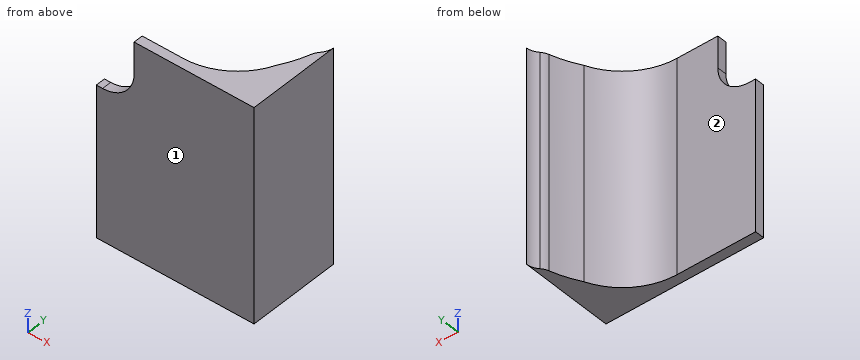
```python
from build123d import *

# Parameters (mm, degrees)
BOSS_EXTRUDE1_DEPTH = 68
CUT_EXTRUDE1_DEPTH  = 10


with BuildPart() as part:
    # Sketch2 → Boss-Extrude1 (new body)
    with BuildSketch(Plane.XY):
        with BuildLine():
            Line((-46.657067634, -11.60759921), (-71.613281954, -11.60759921))
            Line((-71.613281954, -11.60759921), (-71.613281954, -14.607279662))
            Line((-71.613281954, -14.607279662), (-21.613281954, -14.607279662))
            Line((-21.613281954, -14.607279662), (-21.613281954, 15.004436623))
            ThreePointArc((-21.613281954, 15.004436623), (-21.964992236, 13.162317544), (-22.970643034, 11.579355354))
            ThreePointArc((-22.970643034, 11.579355354), (-23.673981627, 10.626616994), (-24.133529038, 9.535190525))
            ThreePointArc((-24.133529038, 9.535190525), (-25.71874065, 5.128724796), (-27.866056136, 0.967129876))
            ThreePointArc((-27.866056136, 0.967129876), (-35.351914775, -8.173910524), (-46.657067634, -11.60759921))
        make_face()
    extrude(amount=BOSS_EXTRUDE1_DEPTH)

    # Sketch3 → Cut-Extrude1 (cut)
    with BuildSketch(Plane(origin=(0, -14.607279662, 0), x_dir=(-1, 0, 0), z_dir=(0, -1, 0))):
        with BuildLine():
            Line((71.613281954, -68), (59.613281954, -68))
            Line((59.613281954, -68), (59.613281954, -58))
            ThreePointArc((59.613281954, -58), (62.542214142, -50.928932188), (69.613281954, -48))
            Line((69.613281954, -48), (71.613281954, -48))
            Line((71.613281954, -48), (71.613281954, -68))
        make_face()
    extrude(amount=-CUT_EXTRUDE1_DEPTH, mode=Mode.SUBTRACT)


solid = part.part
```
Verification items for the finished model (mm, model axes). Face numbers are marked on the shaded views. A direction names the side the tool comes from. Coordinates: 2 decimals unless noted, no trailing zeros. Loops run counter-clockwise (first coordinate to the right, second up) from the corner with the lowest first, then second, coordinate; pieces in that order, holes last. Notation, with made-up numbers: (30, -20.5) -> (40, -20.5) arc R21 cw to (40, -14.5) -> close; hole circle Ø6 at (54.25, 28). An arc over 180 degrees is marked (long way). Answer in a Markdown table with one row per item. Add a question column.
1. Access from +Z, -Z, +X, -X, +Y, -Y to the whole of each face (thin tool, end or side, straight path). Record for the marked faces 1 and 2.
2. Section check A-A, the plane z = 49. Enter the section's corners in (x, y).
3. Section check D-D, the plane z = 8. Enter the section's corners in (x, y).
4. Section check B-B, the plane x = -55.5. Enter the section's corners in (y, z), then the cut area to 3 significant figures.
5. Depth check by flat-ended pin: P1, Ø12, axis at x = -66, z = 40, coming from the +Y side; P2, Ø1.5, axis at y = -7.5, z = 22.5, coming from the -X side; P3, Ø1.6, axis at x = -70.5, y = -12.5, coming from the +Z side. Enter the tip coordinate at first touch or a pass-through.
6. Section check C-C, the plane y = 1.75. Enter the section's corners in (x, z).
7. Material ranges on probe 1 along Y at (x, z) = (-55, 6.5); probe 2 along X at (y, z) = (-10, 34); probe 3 along X at (y, z) = (1, 22.5), recorded low to high. Write a range as [from, to].
Derived:
| question | item | result |
|---|---|---|
| 1 | face 1 | +Z, -Z, +X, -X, -Y |
| 1 | face 2 | +Z, -Z, -X, +Y |
| 2 | outline | (-65.25, -14.61) -> (-21.61, -14.61) -> (-21.61, 15) arc R5 cw to (-22.97, 11.58) arc R5 ccw to (-24.13, 9.54) arc R35.77 cw to (-27.87, 0.97) arc R20.33 cw to (-46.66, -11.61) -> (-65.25, -11.61) -> close |
| 3 | outline | (-71.61, -14.61) -> (-21.61, -14.61) -> (-21.61, 15) arc R5 cw to (-22.97, 11.58) arc R5 ccw to (-24.13, 9.54) arc R35.77 cw to (-27.87, 0.97) arc R20.33 cw to (-46.66, -11.61) -> (-71.61, -11.61) -> close |
| 4 | outline | (-14.61, 0) -> (-11.61, 0) -> (-11.61, 68) -> (-14.61, 68) -> close |
| 4 | area | 204 mm² |
| 5 | P1 | stops at y = -11.61 |
| 5 | P2 | stops at x = -35.47 |
| 5 | P3 | stops at z = 48 |
| 6 | outline | (-27.41, 0) -> (-21.61, 0) -> (-21.61, 68) -> (-27.41, 68) -> close |
| 7 | probe 1 | y = [-14.61, -11.61] |
| 7 | probe 2 | x = [-38.73, -21.61] |
| 7 | probe 3 | x = [-27.85, -21.61] |
